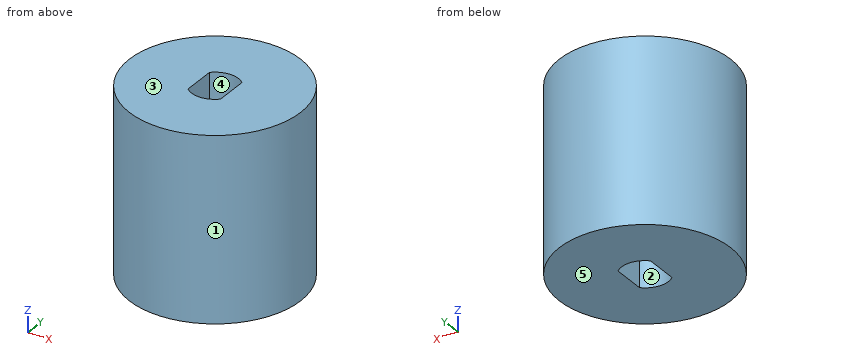
from build123d import *

# Parameters (mm, degrees)
CROQUIS1_R              = 9.85
SALIENTE_EXTRUIR2_DEPTH = 21
CORTAR_EXTRUIR1_DEPTH   = 21


with BuildPart() as part:
    # Croquis1 → Saliente-Extruir2 (new body)
    with BuildSketch(Plane.XY):
        with Locations(Location((0, 0, 0), (0, 0, 180))):
            Circle(CROQUIS1_R)
    extrude(amount=SALIENTE_EXTRUIR2_DEPTH)

    # Croquis2 → Cortar-Extruir1 (cut)
    with BuildSketch(Plane.XY):
        with BuildLine():
            Line((-1.87, 1.947588252), (-1.87, -1.947588252))
            ThreePointArc((-1.87, -1.947588252), (0, -2.7), (1.87, -1.947588252))
            Line((1.87, -1.947588252), (1.87, 1.947588252))
            ThreePointArc((1.87, 1.947588252), (0, 2.7), (-1.87, 1.947588252))
        make_face()
    extrude(amount=CORTAR_EXTRUIR1_DEPTH, mode=Mode.SUBTRACT)


solid = part.part
Work out the finished part from the listing and answer in its coordinate system (mm). Face numbers are marked on the shaded views. A direction names the side the tool comes from. Round coordinates to 2 decimals unless told otherwise and drop trailing zeros. Write each loop counter-clockwise with the first axis right and the second up, starting at its lowest first coordinate (ties: lowest second). Pieces come first, ordered by that corner, then holes. Notation, with made-up numbers: (-20, 31.5) -> (15, 31.5) arc R31 ccw to (15, 59.5) -> close; hole circle Ø11 at (29.5, -0.75). An arc over 180 degrees is marked (long way). Write each question's results on one line, items separated by ' | '.
Item 1: Which of the six approach directions +Z, -Z, +X, -X, +Y, -Y give full straight-line access (tool end or side, diameter ignored) to the marked faces 4 and 5?
Result set:
face 4: +Z, -Z | face 5: -Z, +X, -X, +Y, -Y
Item 2: Find the intervals of material crossed by line 1 along Y through (x, z) = (-1.75, 11); line 2 along X through (y, z) = (1.5, 19.75); line 3 along Y through (x, z) = (8, 17), in increasing order. Write a range as [from, to].
Result set:
line 1: [-9.69, -2.06], [2.06, 9.69] | line 2: [-9.74, -1.87], [1.87, 9.74] | line 3: [-5.75, 5.75]
Item 3: A cutting plane is placed at C-C, the plane z = 6.75. Determine the outline of the cut face in (x, y).
Result set:
outline: circle Ø19.7 at (0, 0); hole (-1.87, -1.95) arc R2.7 ccw to (1.87, -1.95) -> (1.87, 1.95) arc R2.7 ccw to (-1.87, 1.95) -> close
Item 4: A cutting plane is placed at A-A, the plane x = 0. Determine the outline of the cut face in (y, z).
Result set:
outline: (-9.85, 0) -> (-2.7, 0) -> (-2.7, 21) -> (-9.85, 21) -> close; (2.7, 0) -> (9.85, 0) -> (9.85, 21) -> (2.7, 21) -> close
Item 5: A cutting plane is placed at D-D, the plane y = 5.5. Determine the outline of the cut face in (x, z), plus the area to 3 significant figures.
Result set:
outline: (-8.17, 0) -> (8.17, 0) -> (8.17, 21) -> (-8.17, 21) -> close | area: 343 mm^2
Item 6: A cutting plane is placed at B-B, the plane y = 0. Determine the outline of the cut face in (x, z).
Result set:
outline: (-9.85, 0) -> (-1.87, 0) -> (-1.87, 21) -> (-9.85, 21) -> close; (1.87, 0) -> (9.85, 0) -> (9.85, 21) -> (1.87, 21) -> close
Item 7: The mould has two halves that part along Y. Classify the marked faces 1, 2 and 3: +Y half, -Y half, draft (parallel to the pull), parting line (faces both ways), or undercut.
Result set:
face 1: parting line | face 2: undercut | face 3: draft
Item 8: Flat-ended cylindrical pins translate along their axes: P1, Ø5, axis at x = 6.5, z = 3.5, coming from the -Y side; P2, Ø1.5, axis at x = -2.5, z = 17, coming from the +Y side; P3, Ø4, axis at x = -5, z = 5.5, coming from the +Y side. Find the tip coordinate at first contact, or state that the pin passes through.
Result set:
P1: y = -9 | P2: y = 9.69 | P3: y = 9.38
